The model under review builds one solid part; all positions refer to its coordinate system, in mm. Round coordinates to 2 decimals unless told otherwise and drop trailing zeros. Order: outer loops, then holes, each group sorted by start corner. A loop starts at its lowest first (then second) coordinate and runs counter-clockwise, first axis right, second up. Notation, with made-up numbers: M 33.5,-10 L 64.5,-10 A36 cw 64.5,27 Z; hole C 2.5,55 d5. An arc over 180 degrees is marked long. Use a Markdown table: item, result. Add a question column.
1. Consider section A-A on x = 0. State the section outline as (y, z) points (3 decimals), then the cut area to 3 significant figures.
2. Insertion check: P1, Ø1, axis at x = -17.5, z = 4, coming from the +Y side; P2, Ø4, axis at x = 0, y = -25.4, coming from the +Z side. Each pin has a flat end and moves straight along its axis. Give the tip position at first contact, or say it passes through.
3. The part is to be moulded in two halves that separate along Y. For faces 1 (the cylindrical face through (-28.53, -9.18, 2.2)), 2 (the flat face through (-7, 7, 0)), 3 (the cylindrical face through (1.372, 27.552, 2.191)), say which applies: +Y half, -Y half, draft (parallel to the pull), parting line (faces both ways), or undercut.
4. Consider section B-B on z = 2.2. Count the separate pieces of the cut face and the enclosed holes in it, then the cut area to 3 significant figures.
5. To check wall thickness, follow probe 1 along Y at (x, z) = (0, 2.6) (3 decimals); probe 2 along Y at (x, z) = (-27, 0.65); probe 3 along X at (y, z) = (-26, 2.2). State the ranges of each line that lie inside material, in increasing order.
from build123d import *

# Parameters (mm, degrees)
SKETCH1_R           = 2.5527
SKETCH1_R_2         = 9.525
BOSS_EXTRUDE1_DEPTH = 4.445
CHAMFER1_SIZE       = 0.79375
CHAMFER2_SIZE       = 0.79375


with BuildPart() as part:
    # Sketch1 → Boss-Extrude1 (new body)
    with BuildSketch(Plane.XY):
        with BuildLine():
            ThreePointArc((29.827123218, -2.94338318), (17.602792019, 6.406892335), (20.956931757, 21.427267566))
            ThreePointArc((20.956931757, 21.427267566), (-28.16446723, -10.251027736), (29.827123218, -2.94338318))
        make_face()
        with Locations((0, -25.4)):
            Circle(SKETCH1_R, mode=Mode.SUBTRACT)
        with Locations((-25.4, 0)):
            Circle(SKETCH1_R, mode=Mode.SUBTRACT)
        Circle(SKETCH1_R_2, mode=Mode.SUBTRACT)
        with Locations((0, 25.4)):
            Circle(SKETCH1_R, mode=Mode.SUBTRACT)
    extrude(amount=BOSS_EXTRUDE1_DEPTH)

    # Chamfer1
    chamfer1_edges = [part.edges().sort_by_distance(p)[0] for p in [
        (17.602792019, 6.406892335, 4.445),
        (-28.16446723, -10.251027736, 4.445),
    ]]
    chamfer(chamfer1_edges, length=CHAMFER1_SIZE)

    # Chamfer2
    chamfer2_edges = [part.edges().sort_by_distance(p)[0] for p in [
        (-28.16446723, -10.251027736, 0),
        (17.602792019, 6.406892335, 0),
    ]]
    chamfer(chamfer2_edges, length=CHAMFER2_SIZE)


solid = part.part
Answer block:
| question | item | result |
|---|---|---|
| 1 | outline | M -29.972,0.794 L -29.178,0 L -27.953,0 L -27.953,4.445 L -29.178,4.445 L -29.972,3.651 Z; M -22.847,0 L -9.525,0 L -9.525,4.445 L -22.847,4.445 Z; M 9.525,0 L 22.847,0 L 22.847,4.445 L 9.525,4.445 Z; M 27.953,0 L 29.178,0 L 29.972,0.794 L 29.972,3.651 L 29.178,4.445 L 27.953,4.445 Z |
| 1 | area | 135 mm^2 |
| 2 | P1 | y = 24.59 |
| 2 | P2 | through |
| 3 | face 1 | parting line |
| 3 | face 2 | draft |
| 3 | face 3 | undercut |
| 4 | separate pieces | 1 |
| 4 | enclosed holes | 4 |
| 4 | area | 2,270 mm^2 |
| 5 | probe 1 | -29.972 to -27.953, -22.847 to -9.525, 9.525 to 22.847, 27.953 to 29.972 |
| 5 | probe 2 | -12.68 to -1.99, 1.99 to 12.68 |
| 5 | probe 3 | -14.91 to -2.48, 2.48 to 14.91 |
